Geometry: final body of the model. Coordinates: model frame, mm. A direction names the side the tool comes from. Give positions to 0.01 mm unless a question says otherwise; leave off trailing zeros. Write each loop counter-clockwise with the first axis right and the second up, starting at its lowest first coordinate (ties: lowest second). Pieces come first, ordered by that corner, then holes. Notation, with made-up numbers: M 55,11 L 61,11 A27 cw 61,33 Z; hole C -23.75,-22.75 d11. An arc over 180 degrees is marked long. Answer as a JSON object with one key per item and string values.
from build123d import *
from OCP.BRepAlgoAPI import BRepAlgoAPI_Cut
from OCP.TopTools import TopTools_ListOfShape

# Parameters (mm, degrees)
BOSS_EXTRUDE1_DEPTH = 30
SKETCH3_W           = 4
SKETCH3_H           = 15
BOSS_EXTRUDE2_DEPTH = 10
SKETCH4_W           = 4
SKETCH4_H           = 15
CUT_EXTRUDE1_DEPTH  = 35
SKETCH5_R           = 2
CUT_EXTRUDE2_DEPTH  = 35


with BuildPart() as part:
    # Sketch2 → Boss-Extrude1 (new body)
    with BuildSketch(Plane(origin=(0, 0, 0), x_dir=(1, 0, 0), z_dir=(0, 1, 0))):
        with BuildLine():
            Line((0, 12.500000186), (-13.300000086, 12.500000186))
            ThreePointArc((-13.300000086, 12.500000186), (-14.714213649, 11.914213749), (-15.300000086, 10.500000186))
            Line((-15.300000086, 10.500000186), (-15.300000086, 2.350000088))
            Line((-15.300000086, 2.350000088), (-13.646409847, 2.350000088))
            Line((-13.646409847, 2.350000088), (-13.299999759, 2.95))
            Line((-13.299999759, 2.95), (-9.499999695, 2.95))
            Line((-9.499999695, 2.95), (-9.499999695, -2.95))
            Line((-9.499999695, -2.95), (-13.299999759, -2.95))
            Line((-13.299999759, -2.95), (-13.646409847, -2.350000088))
            Line((-13.646409847, -2.350000088), (-15.300000086, -2.350000088))
            Line((-15.300000086, -2.350000088), (-15.300000086, -10.500000186))
            ThreePointArc((-15.300000086, -10.500000186), (-14.714213649, -11.914213749), (-13.300000086, -12.500000186))
            Line((-13.300000086, -12.500000186), (0, -12.500000186))
            Line((0, -12.500000186), (0, 12.500000186))
        make_face()
        with BuildLine():
            Line((13.300000086, 12.500000186), (0, 12.500000186))
            Line((0, 12.500000186), (0, -12.500000186))
            Line((0, -12.500000186), (13.300000086, -12.500000186))
            ThreePointArc((13.300000086, -12.500000186), (14.714213649, -11.914213749), (15.300000086, -10.500000186))
            Line((15.300000086, -10.500000186), (15.300000086, -2.350000088))
            Line((15.300000086, -2.350000088), (13.646408916, -2.350000088))
            Line((13.646408916, -2.350000088), (13.299999759, -2.95))
            Line((13.299999759, -2.95), (9.499998763, -2.95))
            Line((9.499998763, -2.95), (9.499998763, 2.95))
            Line((9.499998763, 2.95), (13.299999759, 2.95))
            Line((13.299999759, 2.95), (13.646408916, 2.350000088))
            Line((13.646408916, 2.350000088), (15.300000086, 2.350000088))
            Line((15.300000086, 2.350000088), (15.300000086, 10.500000186))
            ThreePointArc((15.300000086, 10.500000186), (14.714213649, 11.914213749), (13.300000086, 12.500000186))
        make_face()
    extrude(amount=BOSS_EXTRUDE1_DEPTH)

    # Sketch3 → Boss-Extrude2 (add)
    # profile 1 of 2: a face of its own
    with BuildSketch(Plane(origin=(0, 30, 0), x_dir=(1, 0, 0), z_dir=(0, 1, 0))):
        with BuildLine():
            Line((-9.499999695, 2.95), (-9.499999695, 0))
            Line((-9.499999695, 0), (-9.499999695, -2.95))
            Line((-9.499999695, -2.95), (-9.499999695, -10.000000186))
            ThreePointArc((-9.499999695, -10.000000186), (-8.767766647, -11.767767139), (-6.999999695, -12.500000186))
            Line((-6.999999695, -12.500000186), (6.999999695, -12.500000186))
            ThreePointArc((6.999999695, -12.500000186), (8.767766647, -11.767767139), (9.499999695, -10.000000186))
            Line((9.499999695, -10.000000186), (9.499999695, -2.95))
            Line((9.499999695, -2.95), (9.499999695, 0))
            Line((9.499999695, 0), (9.499999695, 2.95))
            Line((9.499999695, 2.95), (9.499999695, 10.000000186))
            ThreePointArc((9.499999695, 10.000000186), (8.767766647, 11.767767139), (6.999999695, 12.500000186))
            Line((6.999999695, 12.500000186), (-6.999999695, 12.500000186))
            ThreePointArc((-6.999999695, 12.500000186), (-8.767766647, 11.767767139), (-9.499999695, 10.000000186))
            Line((-9.499999695, 10.000000186), (-9.499999695, 2.95))
        make_face()
        with BuildLine():
            Line((4, -9.5), (-4, -9.5))
            ThreePointArc((-4, -9.5), (-5.414213562, -8.914213562), (-6, -7.5))
            Line((-6, -7.5), (-6, 7.5))
            ThreePointArc((-6, 7.5), (-5.414213562, 8.914213562), (-4, 9.5))
            Line((-4, 9.5), (4, 9.5))
            ThreePointArc((4, 9.5), (5.414213562, 8.914213562), (6, 7.5))
            Line((6, 7.5), (6, -7.5))
            ThreePointArc((6, -7.5), (5.414213562, -8.914213562), (4, -9.5))
        make_face(mode=Mode.SUBTRACT)
    # profile 2 of 2: a face of its own
    with BuildSketch(Plane(origin=(0, 30, 0), x_dir=(1, 0, 0), z_dir=(0, 1, 0))):
        with BuildLine():
            ThreePointArc((-6, 7.5), (-5.414213562, 8.914213562), (-4, 9.5))
            Line((-4, 9.5), (4, 9.5))
            ThreePointArc((4, 9.5), (5.414213562, 8.914213562), (6, 7.5))
            Line((6, 7.5), (6, -7.5))
            ThreePointArc((6, -7.5), (5.414213562, -8.914213562), (4, -9.5))
            Line((4, -9.5), (-4, -9.5))
            ThreePointArc((-4, -9.5), (-5.414213562, -8.914213562), (-6, -7.5))
            Line((-6, -7.5), (-6, 7.5))
        make_face()
        Rectangle(SKETCH3_W, SKETCH3_H, mode=Mode.SUBTRACT)
    extrude(amount=BOSS_EXTRUDE2_DEPTH)

    # Sketch4 → Cut-Extrude1 (cut)
    with BuildSketch(Plane(origin=(0, 40, 0), x_dir=(1, 0, 0), z_dir=(0, 1, 0))):
        Rectangle(SKETCH4_W, SKETCH4_H)
    extrude(amount=-CUT_EXTRUDE1_DEPTH, mode=Mode.SUBTRACT)


with BuildPart() as cut_extrude2_tool:
    # Sketch5 → Cut-Extrude2 (new body)
    with BuildSketch(Plane(origin=(9.499998763, 0, 0), x_dir=(0, 0, -1), z_dir=(1, 0, 0))):
        with Locations((5, 35)):
            Circle(SKETCH5_R)
        with Locations((0, 35)):
            Circle(SKETCH5_R)
        with Locations((-5, 35)):
            Circle(SKETCH5_R)
    extrude(amount=-CUT_EXTRUDE2_DEPTH)


with BuildPart() as part_1:
    add(part.part)

    # Cut-Extrude2: cut by cut_extrude2_tool, with a tolerance
    cut_extrude2_stock = TopTools_ListOfShape()
    cut_extrude2_stock.Append(part_1.part.wrapped)
    cut_extrude2_tools = TopTools_ListOfShape()
    cut_extrude2_tools.Append(cut_extrude2_tool.part.wrapped)
    cut_extrude2_cut = BRepAlgoAPI_Cut()
    cut_extrude2_cut.SetArguments(cut_extrude2_stock)
    cut_extrude2_cut.SetTools(cut_extrude2_tools)
    cut_extrude2_cut.SetFuzzyValue(0.00001)
    cut_extrude2_cut.Build()
    add(Compound.cast(cut_extrude2_cut.Shape()).solids(), mode=Mode.REPLACE)


solid = part_1.part
1) Line query: line 1 (X direction, y = 24, z = 5); line 2 (Z direction, x = 12, y = 23.5); line 3 (Y direction, x = -5.5, z = 5). Output: solid intervals per line, ascending. Write a range as from..to.
Geometry check:
{"line 1": "x = -15.3..-2, 2..15.3", "line 2": "z = -12.5..-2.95, 2.95..12.5", "line 3": "y = 0..33, 37..40"}
2) Cut plane A-A on x = 11.5. Return loops of the section in (y, z).
Geometry check:
{"outline": "M 0,-12.5 L 30,-12.5 L 30,-2.95 L 0,-2.95 Z; M 0,2.95 L 30,2.95 L 30,12.5 L 0,12.5 Z"}
3) Pull-direction query (X, two-part tool) for faces 1 (the cylindrical face through (8.748, 34.93, 11.787)), 2 (the flat face through (0, 22, 7.5)), 3 (the cylindrical face through (6, 33, -5)); classes: pulls with the +X half, pulls with the -X half, needs draft (parallel to the pull), parting line crosses it, or undercut.
Geometry check:
{"face 1": "pulls with the +X half", "face 2": "undercut", "face 3": "needs draft"}
4) Set-up query: faces 4 (the cylindrical face through (-8.787, 34.93, 11.748)), 5 (the flat face through (14, 15, -2.35)), 6 (the flat face through (-14, 15, 2.35)), 7 (the flat face through (11, 15, 2.95)). Return all of +Z, -Z, +X, -X, +Y, -Y with unobstructed straight access to the full face (end or side cutting, diameter ignored); none if empty.
Geometry check:
{"face 4": "+Z, -X, +Y", "face 5": "+X, +Y, -Y", "face 6": "-X, +Y, -Y", "face 7": "+Y, -Y"}
5) Cut plane C-C on y = 7. Return loops of the section in (x, z), and give its area (3 significant figures).
Geometry check:
{"outline": "M -15.3,-10.5 A2 ccw -13.3,-12.5 L 13.3,-12.5 A2 ccw 15.3,-10.5 L 15.3,-2.35 L 13.65,-2.35 L 13.3,-2.95 L 9.5,-2.95 L 9.5,2.95 L 13.3,2.95 L 13.65,2.35 L 15.3,2.35 L 15.3,10.5 A2 ccw 13.3,12.5 L -13.3,12.5 A2 ccw -15.3,10.5 L -15.3,2.35 L -13.65,2.35 L -13.3,2.95 L -9.5,2.95 L -9.5,-2.95 L -13.3,-2.95 L -13.65,-2.35 L -15.3,-2.35 Z; hole M -2,-7.5 L 2,-7.5 L 2,7.5 L -2,7.5 Z", "area": "638 mm2"}
6) Cut plane B-B on z = 0. Give the number of separate pieces and of enclosed holes in the cut face, and give its area (3 significant figures).
Geometry check:
{"separate pieces": "3", "enclosed holes": "0", "area": "560 mm2"}
7) Contact query for flat-ended pins moving along their axis: P1, Ø5, axis at y = 35, z = -5, coming from the +X side; P2, Ø1, axis at x = 12, z = 4, coming from the +Y side; P3, Ø1.2, axis at x = -1, z = 3.5, coming from the +Y side. Output: stop coordinate, or through.
Geometry check:
{"P1": "stops at x = 9.5", "P2": "stops at y = 30", "P3": "stops at y = 5"}
8) Cut plane D-D on x = 3. Return loops of the section in (y, z), and give its area (3 significant figures).
Geometry check:
{"outline": "M 0,-12.5 L 40,-12.5 L 40,12.5 L 0,12.5 Z; hole C 35,-5 d4; hole C 35,0 d4; hole C 35,5 d4", "area": "962 mm2"}
